from build123d import *

# Parameters (mm, degrees)
SKETCH_1_W          = 34
SKETCH_1_H          = 30
SKETCH_1_R          = 2.6
EXTRUDE_1_DEPTH     = 2
SKETCH_2_R          = 1.75
CUT_EXTRUDE_1_DEPTH = 2
SKETCH_3_W          = 10
SKETCH_3_H          = 10
CUT_EXTRUDE_2_DEPTH = 2
FILLET_1_R          = 2


with BuildPart() as part:
    # 草图1 → 凸台-拉伸1 (new body)
    with BuildSketch(Plane.XY):
        Rectangle(SKETCH_1_W, SKETCH_1_H)
        Circle(SKETCH_1_R, mode=Mode.SUBTRACT)
    extrude(amount=EXTRUDE_1_DEPTH)

    # 草图2 → 切除-拉伸1 (cut)
    with BuildSketch(Plane(origin=(0, 0, 0), x_dir=(-1, 0, 0), z_dir=(0, 0, -1))):
        with Locations((10.5, -10.5)):
            Circle(SKETCH_2_R)
        with Locations((-10.5, -10.5)):
            Circle(SKETCH_2_R)
        with Locations((-10.5, 10.5)):
            Circle(SKETCH_2_R)
        with Locations((10.5, 10.5)):
            Circle(SKETCH_2_R)
    extrude(amount=-CUT_EXTRUDE_1_DEPTH, mode=Mode.SUBTRACT)

    # 草图3 → 切除-拉伸2 (cut)
    with BuildSketch(Plane.XY.offset(2)):
        with Locations((-12, 0)):
            Rectangle(SKETCH_3_W, SKETCH_3_H)
        with Locations((0, 12)):
            Rectangle(SKETCH_3_W, SKETCH_3_H)
        with Locations((12, 0)):
            Rectangle(SKETCH_3_W, SKETCH_3_H)
        with Locations((0, -12)):
            Rectangle(SKETCH_3_W, SKETCH_3_H)
    extrude(amount=-CUT_EXTRUDE_2_DEPTH, mode=Mode.SUBTRACT)

    # 圆角1
    fillet_1_edges = [part.edges().sort_by_distance(p)[0] for p in [
        (-17, -5, 1),
        (-17, 5, 1),
        (-7, 5, 1),
        (-7, -5, 1),
        (-5, 15, 1),
        (5, 15, 1),
        (-5, 7, 1),
        (5, 7, 1),
        (17, -5, 1),
        (7, -5, 1),
        (7, 5, 1),
        (17, 5, 1),
        (17, -15, 1),
        (-17, -15, 1),
        (-17, 15, 1),
        (17, 15, 1),
        (5, -15, 1),
        (-5, -15, 1),
        (5, -7, 1),
        (-5, -7, 1),
    ]]
    fillet(fillet_1_edges, radius=FILLET_1_R)


solid = part.part
Geometry check sheet. Reference: the model listing, model coordinates, mm. A direction names the side the tool comes from. Round coordinates to 2 decimals unless told otherwise and drop trailing zeros. Order: outer loops, then holes, each group sorted by start corner. A loop starts at its lowest first (then second) coordinate and runs counter-clockwise, first axis right, second up. Notation, with made-up numbers: M -30.5,-18 L -14.5,-18 A29 ccw -14.5,9 Z; hole C 20,15.5 d11. An arc over 180 degrees is marked long. Answer in a Markdown table with one row per item.
(1) Scan lines: probe 1 along Y at (x, z) = (10.5, 1.55); probe 2 along Y at (x, z) = (0, 0.5); probe 3 along Y at (x, z) = (12.5, 0.35). Record each from-to range of solid material in increasing order. Write a range as from..to.
Responses:
| item | result |
|---|---|
| probe 1 | y = -15..-12.25, -8.75..-5, 5..8.75, 12.25..15 |
| probe 2 | y = -7..-2.6, 2.6..7 |
| probe 3 | y = -15..-5, 5..15 |
(2) Sectioned sample at D-D, the plane z = 0.85. State how many separate pieces and enclosed holes the cut face has, and give its area (3 significant figures).
Responses:
| item | result |
|---|---|
| separate pieces | 1 |
| enclosed holes | 5 |
| area | 597 mm² |
(3) Sectioned sample at B-B, the plane y = -10.5. Record the cut outline in (x, z).
Responses:
| item | result |
|---|---|
| outline | M -17,0 L -12.25,0 L -12.25,2 L -17,2 Z; M -8.75,0 L -5,0 L -5,2 L -8.75,2 Z; M 5,0 L 8.75,0 L 8.75,2 L 5,2 Z; M 12.25,0 L 17,0 L 17,2 L 12.25,2 Z |
(4) Sectioned sample at C-C, the plane y = 0. Record the cut outline in (x, z), and give its area (3 significant figures).
Responses:
| item | result |
|---|---|
| outline | M -7,0 L -2.6,0 L -2.6,2 L -7,2 Z; M 2.6,0 L 7,0 L 7,2 L 2.6,2 Z |
| area | 17.6 mm² |
(5) Tool access check on faces 1 (the face through (16.43, -14.4, 1.01)), 2 (the face through (-7.6, -4.43, 0.99)), 3 (the face through (11, -15, 1)), 4 (the face through (0, 7, 1)), 5 (the face through (12, 5, 1)). Record the directions out of +Z, -Z, +X, -X, +Y, -Y that give a thin tool (end or side, any length) a straight path to the whole face; none if there is none.
Responses:
| item | result |
|---|---|
| face 1 | +Z, -Z, +X, -Y |
| face 2 | +Z, -Z, -X |
| face 3 | +Z, -Z, +X, -X, -Y |
| face 4 | +Z, -Z, +Y |
| face 5 | +Z, -Z, +X |
(6) Sectioned sample at A-A, the plane x = -14. Record the cut outline in (y, z), and give its area (3 significant figures).
Responses:
| item | result |
|---|---|
| outline | M -15,0 L -5,0 L -5,2 L -15,2 Z; M 5,0 L 15,0 L 15,2 L 5,2 Z |
| area | 40.0 mm² |
(7) Go/stop test with a flat-tipped pin: P1, Ø4, axis at x = 13, y = 2, coming from the +Z side. Record where the tip stops, or that it passes through.
Responses:
| item | result |
|---|---|
| P1 | passes through |
(8) Draft check along X on faces 6 (the face through (9.6, 12, 1)), 7 (the face through (5.57, 14.4, 0.99)), 8 (the face through (17, -10, 1)), 9 (the face through (-11, -15, 1)). Enter one of: released by +X, released by -X, zero draft, split by the parting line, or undercut.
Responses:
| item | result |
|---|---|
| face 6 | undercut |
| face 7 | undercut |
| face 8 | released by +X |
| face 9 | zero draft |
